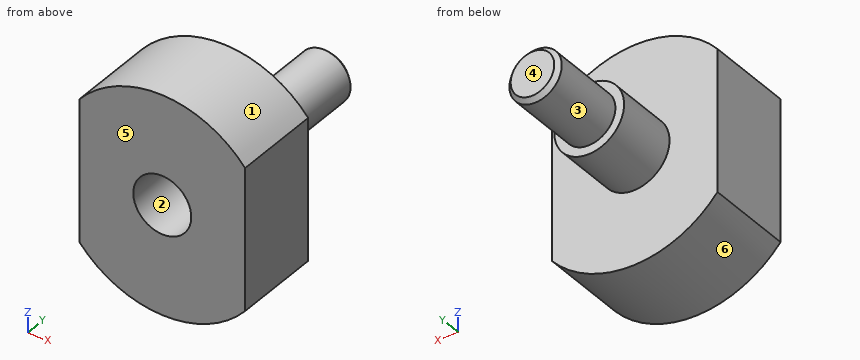
Autodesk Inventor part; units mm, degrees
ref_plane "YZ Plane" through (0, 0, 0) normal (1, 0, 0) x (0, 1, 0)
ref_plane "XZ Plane" through (0, 0, 0) normal (0, 1, 0) x (-1, 0, 0)
ref_plane "XY Plane" through (0, 0, 0) normal (0, 0, 1) x (1, 0, 0)
sketch "Sketch1" plane through (0, 0, 0) normal (0, 1, 0) x (-1, 0, 0)
  circle A0 centre (0, 0) radius 12.5
  dimension "d0" = 25
extrude "Extrusion1" add sketch "Sketch1" along normal blind 10
sketch "Sketch2" plane through (0, 10, 0) normal (0, 1, 0) x (1, 0, 0)
  circle A0 centre (0, 0) radius 4
  dimension "d3" = 8
extrude "Extrusion2" add sketch "Sketch2" along normal blind 7.2
sketch "Sketch3" plane through (0, 17.2, 0) normal (0, 1, 0) x (1, 0, 0)
  circle A0 centre (0, 0) radius 4
  circle A1 centre (0, 0) radius 3
  dimension "d6" = 6
extrude "Extrusion3" add sketch "Sketch3" along normal blind 9 contours A1
chamfer "Chamfer1" distance 0.5 angle 45 1 edges at (-3, 26.2, 0)
thread "Thread1"
sketch "Sketch4" plane through (0, 0, 0) normal (0, -1, 0) x (1, 0, 0)
  point P0 (0, 0)
  point P1 (0, 0)
hole "Hole1" at (0, 0, 0) direction (0, 1, 0) diameter 6.647 depth 8 tip angle 118
sketch "Sketch5" plane through (0, 0, 0) normal (0, -1, 0) x (1, 0, 0)
  circle A0 centre (0, 0) radius 12.5
  line L0 (9.5, -8.124) -> (-9.5, -8.124)
  line L1 (-9.5, -8.124) -> (-9.5, 8.124)
  line L2 (-9.5, 8.124) -> (9.5, 8.124)
  line L3 (9.5, 8.124) -> (9.5, -8.124)
  line L4 (9.5, -8.124) -> (-9.5, 8.124) construction
  line L5 (-9.5, -8.124) -> (9.5, 8.124) construction
  dimension "d21" = 19
extrude "Extrusion4" cut sketch "Sketch5" against normal through all contours A0 L3 | L1 A0
properties part number "Fixing Stud Pt 2"
Geometry check sheet. Reference: the model listing, model coordinates, mm. Face numbers are marked on the shaded views. A direction names the side the tool comes from. Give positions to 0.01 mm unless a question says otherwise; leave off trailing zeros. Order: outer loops, then holes, each group sorted by start corner. A loop starts at its lowest first (then second) coordinate and runs counter-clockwise, first axis right, second up. Notation, with made-up numbers: (-24, -32.75) - (-8, -32.75) arc R30 cw to (-8, 2.25) - close; hole circle Ø5 at (-17, 28.25). An arc over 180 degrees is marked (long way). Write item = value, one per line. Start each with the question number.
1) Access from +Z, -Z, +X, -X, +Y, -Y to the whole of each face (thin tool, end or side, straight path). Record for the marked faces 1, 2 and 3.
2) Scan lines: L1, parallel to Z at x = 0, y = 6.5; L2, parallel to X at y = 3, z = 0; L3, parallel to Y at x = -2.25, z = -10.5. Record each from-to range of solid material in increasing order.
3) Section check D-D (x = -5). Enter the section's corners in (y, z), then the cut area to 3 significant figures.
4) Gauge pin test, flat ends, axial feed: pin 1 Ø1.5 at (x, y) = (3.5, 4) entering from +Z; pin 2 Ø5 at (x, y) = (3.5, 7.5) entering from +Z; pin 3 Ø1 at (x, y) = (-4, 22) entering from +Z; pin 4 Ø3 at (x, y) = (-3.5, 9.5) entering from -Z. Record the tip position at first contact, or that the pin passes through.
5) Section check A-A (y = 7.25). Enter the section's corners in (x, z).
6) Draft check along Y on the marked faces 4, 5 and 6. Enter one of: released by +Y, released by -Y, zero draft, split by the parting line, or undercut.
7) Section check C-C (y = 23.5). Enter the section's corners in (x, z), then the cut area to 3 significant figures.
8) Section check B-B (z = 4.5). Enter the section's corners in (x, y), then the cut area to 3 significant figures.
Geometry check:
q1.face_1 = +Z, +Y, -Y
q1.face_2 = -Y
q1.face_3 = +Y
q2.L1 = -12.5 to -3.32, 3.32 to 12.5
q2.L2 = -9.5 to -3.32, 3.32 to 9.5
q2.L3 = 0 to 10
q3.outline = (0, -11.46) - (10, -11.46) - (10, 11.46) - (0, 11.46) - close
q3.area = 229 mm2
q4.pin_1 = 12.19
q4.pin_2 = 12.46
q4.pin_3 = through
q4.pin_4 = -12.34
q5.outline = (-9.5, -8.12) arc R12.5 ccw to (9.5, -8.12) - (9.5, 8.12) arc R12.5 ccw to (-9.5, 8.12) - close; hole circle Ø6.65 at (0, 0)
q6.face_4 = released by +Y
q6.face_5 = released by -Y
q6.face_6 = zero draft
q7.outline = circle Ø6 at (0, 0)
q7.area = 28.3 mm2
q8.outline = (-9.5, 0) - (9.5, 0) - (9.5, 10) - (-9.5, 10) - close
q8.area = 190 mm2
